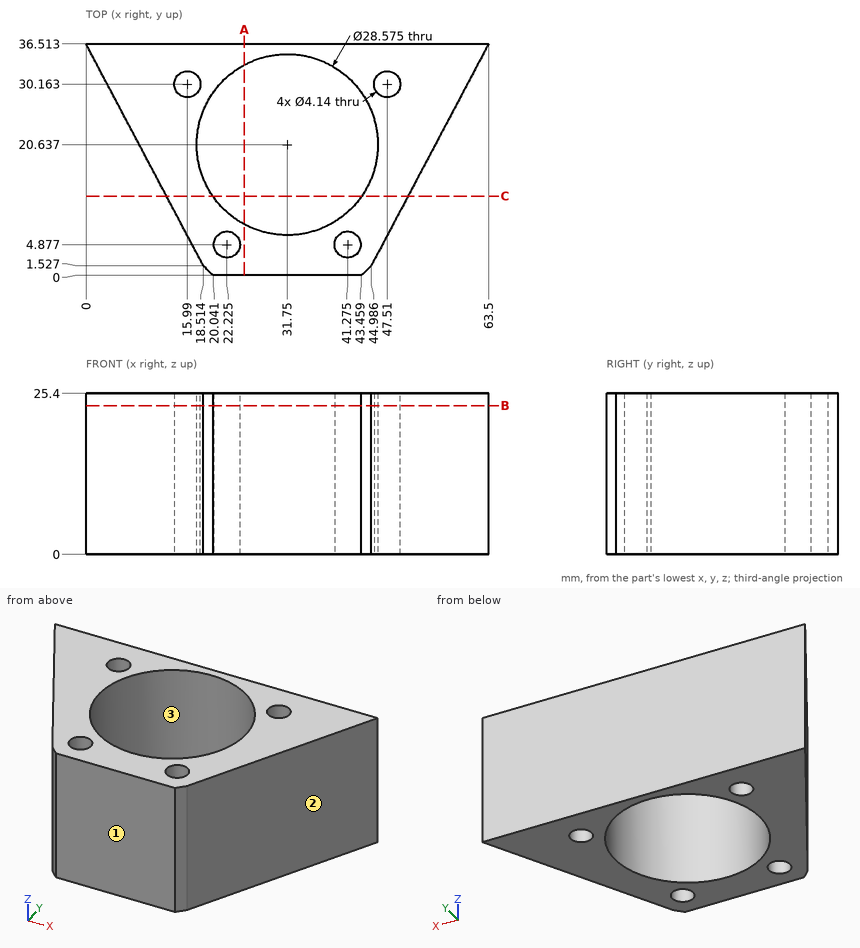
Could you check a few things on this drawing? It's one solid part, dimensions in mm from its lowest x, y, z. Give positions to 0.01 mm unless a question says otherwise; leave off trailing zeros. Loops run counter-clockwise (first coordinate to the right, second up) from the corner with the lowest first, then second, coordinate; pieces in that order, holes last. Notation, with made-up numbers: M 71.5,-7.75 L 101.5,-7.75 A14 cw 101.5,9.25 Z; hole C 77.25,43.25 d1. An arc over 180 degrees is marked long. Answer as a JSON object with one key per item and string values.
Q1. If I drill on probe 1 along X at (y, z) = (30, 23) (1 decimal); probe 2 along Y at (x, z) = (24, 4) (1 decimal); probe 3 along Y at (x, z) = (32, 19.5), over which ranges is the centre line in solid material (lowest first)? Write a range as [from, to].
Values found:
{"probe 1": "x = [3.4, 13.9], [18.1, 21], [42.5, 45.4], [49.6, 60.1]", "probe 2": "y = [0, 3.8], [5.9, 8.6], [32.6, 36.5]", "probe 3": "y = [0, 6.35], [34.92, 36.51]"}
Q2. If we mould it in two halves opening along X, with no side actions, what happens to the marked faces 1, 2 and 3? For each: pulls with the +X half, pulls with the -X half, needs draft (parallel to the pull), parting line crosses it, or undercut.
Values found:
{"face 1": "needs draft", "face 2": "pulls with the +X half", "face 3": "undercut"}
Q3. For P1, Ø1, axis at y = 28, z = 13, coming from the +X side; P2, Ø2.5, axis at x = 47.51, y = 30.16, coming from the -Z side; P3, Ø8, axis at y = 23, z = 8, coming from the +X side (1 decimal); P4, Ø12, axis at x = 54, z = 12.5, coming from the -Y side (1 decimal), each with a flat end and sliding along its axis, tell me the tip position at first contact or that it passes through.
Values found:
{"P1": "stops at x = 59.26", "P2": "passes through", "P3": "stops at x = 58.5", "P4": "stops at y = 7.2"}
Q4. Suppose I cut it at B-B, the plane z = 23.5. State how many separate pieces and enclosed holes the cut face has.
Values found:
{"separate pieces": "1", "enclosed holes": "5"}
Q5. Suppose I cut it at A-A, the plane x = 25. List the corners of the cut face in (y, z) for me (1 decimal), plus the area to 3 significant figures.
Values found:
{"outline": "M 0,0 L 8,0 L 8,25.4 L 0,25.4 Z; M 33.2,0 L 36.5,0 L 36.5,25.4 L 33.2,25.4 Z", "area": "288 mm²"}
Q6. Suppose I cut it at C-C, the plane y = 12.5. List the corners of the cut face in (x, z) for me.
Values found:
{"outline": "M 12.71,0 L 20.01,0 L 20.01,25.4 L 12.71,25.4 Z; M 43.49,0 L 50.79,0 L 50.79,25.4 L 43.49,25.4 Z"}
